from build123d import *

# Parameters (mm, degrees)
CROQUIS1_W              = 400
CROQUIS1_H              = 380
SALIENTE_EXTRUIR1_DEPTH = 95
CROQUIS2_W              = 30.4
CROQUIS2_H              = 21.7
CROQUIS2_W_2            = 1
CROQUIS2_H_2            = 5
CORTAR_EXTRUIR1_DEPTH   = 14
CROQUIS3_W              = 45
CROQUIS3_H              = 150
CROQUIS3_W_2            = 100
CROQUIS3_H_2            = 15
SALIENTE_EXTRUIR2_DEPTH = 3
CROQUIS4_R              = 6.15
CROQUIS4_R_2            = 4
CROQUIS4_W              = 5
CROQUIS4_H              = 13
CROQUIS4_W_2            = 12
SALIENTE_EXTRUIR3_DEPTH = 5
CROQUIS5_R              = 4.1
CROQUIS5_R_2            = 5.55
SALIENTE_EXTRUIR4_DEPTH = 5
CROQUIS6_W              = 160
CROQUIS6_H              = 70
CROQUIS6_W_2            = 43.6
CROQUIS6_H_2            = 6
CROQUIS6_W_3            = 22.5
CROQUIS6_R              = 3
CROQUIS6_W_4            = 13.5
CROQUIS6_H_3            = 8
CROQUIS6_H_4            = 20
CORTAR_EXTRUIR2_DEPTH   = 12.8


with BuildPart() as part:
    # Croquis1 → Saliente-Extruir1 (new body, symmetric)
    with BuildSketch(Plane(origin=(0, 0, 0), x_dir=(0, 0, -1), z_dir=(1, 0, 0))):
        Rectangle(CROQUIS1_W, CROQUIS1_H)
    extrude(amount=SALIENTE_EXTRUIR1_DEPTH, both=True)

    # Croquis2 → Cortar-Extruir1 (cut)
    with BuildSketch(Plane(origin=(0, 0, -200), x_dir=(-1, 0, 0), z_dir=(0, 0, -1))):
        with Locations((-55, 160)):
            Rectangle(CROQUIS2_W, CROQUIS2_H)
        Polygon((-42, 151), (-68, 151), (-68, 160), (-68, 164.669872981), (-62.5, 169), (-47.5, 169), (-42, 164.669872981), (-42, 160), align=None, mode=Mode.SUBTRACT)
        with Locations((-55, 162.856907895)):
            Rectangle(CROQUIS2_W_2, CROQUIS2_H_2)
        with Locations((-48.5, 155)):
            Rectangle(CROQUIS2_W_2, CROQUIS2_H_2)
        with Locations((-61.5, 155)):
            Rectangle(CROQUIS2_W_2, CROQUIS2_H_2)
        Polygon((-85, 90), (-25, 90), (-25, -70), (30, -70), (30, -165), (-85, -165), align=None)
    extrude(amount=-CORTAR_EXTRUIR1_DEPTH, mode=Mode.SUBTRACT)

    # Croquis3 → Saliente-Extruir2 (add)
    with BuildSketch(Plane(origin=(0, 0, -186), x_dir=(-1, 0, 0), z_dir=(0, 0, -1))):
        with Locations((-58, 12.5)):
            Rectangle(CROQUIS3_W, CROQUIS3_H)
        with Locations((-22.5, -85)):
            Rectangle(CROQUIS3_W_2, CROQUIS3_H_2)
    extrude(amount=SALIENTE_EXTRUIR2_DEPTH)

    # Croquis4 → Saliente-Extruir3 (add)
    with BuildSketch(Plane(origin=(0, 0, -189), x_dir=(-1, 0, 0), z_dir=(0, 0, -1))):
        with Locations((-69, 76)):
            Circle(CROQUIS4_R)
        with Locations((-50, 76)):
            Circle(CROQUIS4_R)
        with Locations((-68, -57.5)):
            Circle(CROQUIS4_R_2)
        with Locations((-56, -57.5)):
            Circle(CROQUIS4_R_2)
        with Locations((-43, -57.5)):
            Circle(CROQUIS4_R_2)
        with BuildLine():
            Line((-65.269265107, 53.441675937), (-70.469265107, 52.735154197))
            ThreePointArc((-70.469265107, 52.735154197), (-71.706408015, 52.068936991), (-72.2, 50.753363012))
            Line((-72.2, 50.753363012), (-72.2, 41.246636988))
            ThreePointArc((-72.2, 41.246636988), (-71.706408015, 39.931063009), (-70.469265107, 39.264845803))
            Line((-70.469265107, 39.264845803), (-65.269265107, 38.558324063))
            ThreePointArc((-65.269265107, 38.558324063), (-63.684426021, 39.033707234), (-63, 40.540115249))
            Line((-63, 40.540115249), (-63, 51.459884751))
            ThreePointArc((-63, 51.459884751), (-63.684426021, 52.966292766), (-65.269265107, 53.441675937))
        make_face()
        with BuildLine():
            Line((-52.36857707, 53.105891799), (-48.36857707, 53.855891799))
            ThreePointArc((-48.36857707, 53.855891799), (-46.722728326, 53.429165642), (-46, 51.890147425))
            Line((-46, 51.890147425), (-46, 16.709852575))
            ThreePointArc((-46, 16.709852575), (-46.722728326, 15.170834358), (-48.36857707, 14.744108201))
            Line((-48.36857707, 14.744108201), (-52.36857707, 15.494108201))
            ThreePointArc((-52.36857707, 15.494108201), (-53.539018216, 16.1825809), (-54, 17.459852575))
            Line((-54, 17.459852575), (-54, 51.140147425))
            ThreePointArc((-54, 51.140147425), (-53.539018216, 52.4174191), (-52.36857707, 53.105891799))
        make_face()
        with BuildLine():
            Line((-68.25, 23), (-70, 23))
            Line((-70, 23), (-70, 4))
            Line((-70, 4), (-68.25, 4))
            ThreePointArc((-68.25, 4), (-65, 0.75), (-61.75, 4))
            Line((-61.75, 4), (-60, 4))
            Line((-60, 4), (-60, 23))
            Line((-60, 23), (-61.75, 23))
            ThreePointArc((-61.75, 23), (-65, 26.25), (-68.25, 23))
        make_face()
        with Locations((-63, -13.5)):
            Rectangle(CROQUIS4_W, CROQUIS4_H)
        with Locations((-71, -13.5)):
            Rectangle(CROQUIS4_W, CROQUIS4_H)
        with Locations((-63, -40.5)):
            Rectangle(CROQUIS4_W, CROQUIS4_H)
        with Locations((-71, -40.5)):
            Rectangle(CROQUIS4_W, CROQUIS4_H)
        with BuildLine():
            Line((-46, -20.5), (-46, -6.5))
            Line((-46, -6.5), (-56, -6.5))
            Line((-56, -6.5), (-56, -20.5))
            ThreePointArc((-56, -20.5), (-51, -25.5), (-46, -20.5))
        make_face()
        with Locations((-50, -40.5)):
            Rectangle(CROQUIS4_W_2, CROQUIS4_H)
    extrude(amount=SALIENTE_EXTRUIR3_DEPTH)

    # Croquis5 → Saliente-Extruir4 (add)
    with BuildSketch(Plane(origin=(0, 0, -189), x_dir=(-1, 0, 0), z_dir=(0, 0, -1))):
        with Locations((-13, -85)):
            Circle(CROQUIS5_R)
        with Locations((-28, -85)):
            Circle(CROQUIS5_R_2)
        with BuildLine():
            Line((-54.378732187, -82.51492875), (-55.378732187, -86.51492875))
            ThreePointArc((-55.378732187, -86.51492875), (-55.014858063, -88.230824419), (-53.438447187, -89))
            Line((-53.438447187, -89), (-42.561552813, -89))
            ThreePointArc((-42.561552813, -89), (-40.985141937, -88.230824419), (-40.621267813, -86.51492875))
            Line((-40.621267813, -86.51492875), (-41.621267813, -82.51492875))
            ThreePointArc((-41.621267813, -82.51492875), (-42.330728394, -81.423589124), (-43.561552813, -81))
            Line((-43.561552813, -81), (-52.438447187, -81))
            ThreePointArc((-52.438447187, -81), (-53.669271606, -81.423589124), (-54.378732187, -82.51492875))
        make_face()
    extrude(amount=SALIENTE_EXTRUIR4_DEPTH)

    # Croquis6 → Cortar-Extruir2 (cut)
    with BuildSketch(Plane.XY.offset(200)):
        with Locations((0, 35)):
            Rectangle(CROQUIS6_W, CROQUIS6_H)
        with Locations((-53, 16)):
            Rectangle(CROQUIS6_W_2, CROQUIS6_H_2, mode=Mode.SUBTRACT)
        with Locations((-53, 25)):
            Rectangle(CROQUIS6_W_2, CROQUIS6_H_2, mode=Mode.SUBTRACT)
        with Locations((-8, 16)):
            Rectangle(CROQUIS6_W_3, CROQUIS6_H_2, mode=Mode.SUBTRACT)
        with Locations((-8, 25)):
            Rectangle(CROQUIS6_W_3, CROQUIS6_H_2, mode=Mode.SUBTRACT)
        Polygon((17.5, 58), (17.5, 50), (-12, 50), (-12, 42), (-44, 42), (-44, 50), (-73.5, 50), (-73.5, 58), (-44, 58), (-44, 66), (-12, 66), (-12, 58), align=None, mode=Mode.SUBTRACT)
        with Locations((52, 15)):
            Circle(CROQUIS6_R, mode=Mode.SUBTRACT)
        with Locations((68, 15)):
            Rectangle(CROQUIS6_W_4, CROQUIS6_H_3, mode=Mode.SUBTRACT)
        with Locations((52, 35)):
            Circle(CROQUIS6_R, mode=Mode.SUBTRACT)
        with Locations((52, 55)):
            Circle(CROQUIS6_R, mode=Mode.SUBTRACT)
        with Locations((68, 51)):
            Rectangle(CROQUIS6_W_4, CROQUIS6_H_3, mode=Mode.SUBTRACT)
        with Locations((0, 165)):
            Rectangle(CROQUIS6_W, CROQUIS6_H_4)
        with Locations((0, 125)):
            Rectangle(CROQUIS6_W, CROQUIS6_H_4)
    extrude(amount=-CORTAR_EXTRUIR2_DEPTH, mode=Mode.SUBTRACT)


solid = part.part
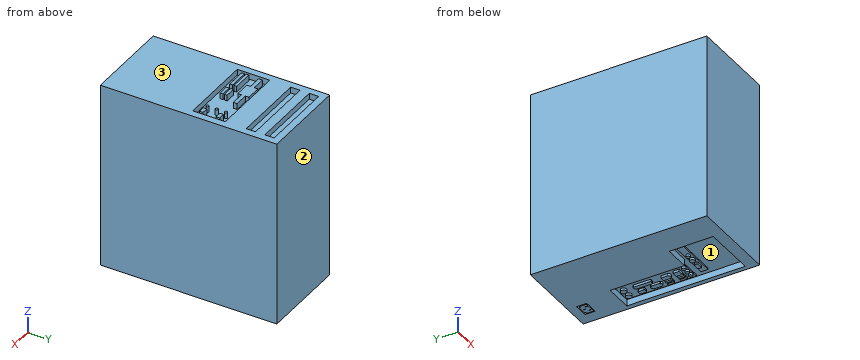
Geometry check sheet. Reference: the model listing, model coordinates, mm. Face numbers are marked on the shaded views. Give positions to 0.01 mm unless a question says otherwise; leave off trailing zeros. Use a Markdown table: item, result.
Item 1: Draft check along Y on the marked faces 1, 2 and 3. Enter one of: +Y half, -Y half, draft (parallel to the pull), parting line (faces both ways), or undercut.
Answers follow:
| item | result |
|---|---|
| face 1 | undercut |
| face 2 | +Y half |
| face 3 | draft |
Item 2: Material ranges on line 1 along Z through (x, y) = (-69.5, 134); line 2 along Z through (x, y) = (17, -114.5), recorded low to high.
Answers follow:
| item | result |
|---|---|
| line 1 | z = -200 to 187.2 |
| line 2 | z = -186 to 200 |
Item 3: Depth check by flat-ended pin: P1, Ø1.5, axis at x = 63, y = -40, coming from the -Z side. Enter the tip coordinate at first touch or a pass-through.
Answers follow:
| item | result |
|---|---|
| P1 | stops at z = -194 |
